Geometry check sheet. Reference: drawing and pictorial views, mm from the part's lowest x, y, z. Give positions to 0.01 mm unless a question says otherwise; leave off trailing zeros. Write each loop counter-clockwise with the first axis right and the second up, starting at its lowest first coordinate (ties: lowest second). Pieces come first, ordered by that corner, then holes. Notation, with made-up numbers: (45, -12) -> (64, -12) arc R21 cw to (64, 25) -> close; hole circle Ø11 at (-12.5, -7.75). An arc over 180 degrees is marked (long way). Write each question's results on one line, items separated by ' | '. Start each with the question number.
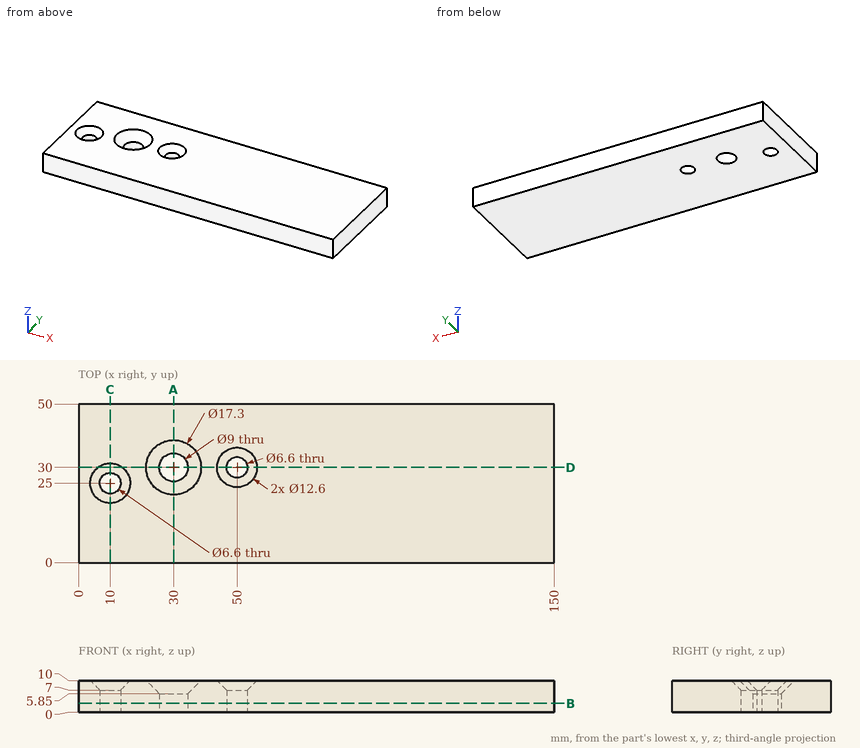
Item 1: Section check B-B on z = 2.75. Record the boundary of the cut face in (x, y).
Item 2: Section check A-A on x = 30. Record the boundary of the cut face in (y, z), then the cut area to 3 significant figures.
Item 3: Section check D-D on y = 30. Count the separate pieces of the cut face and the enclosed holes in it, then the cut area to 3 significant figures.
Item 4: Thickness scan on probe 1 along X at (y, z) = (30, 3.5); probe 2 along Y at (x, z) = (10, 1.5); probe 3 along X at (y, z) = (25, 4.5). Record the ranges inside material, lowest first. Write a range as from..to.
Item 5: Depth check by flat-ended pin: pin 1 Ø5.5 at (x, y) = (30, 30) entering from +Z. Enter the tip coordinate at first touch or a pass-through.
Item 6: Section check C-C on x = 10. Record the boundary of the cut face in (y, z), then the cut area to 3 significant figures.
Check sheet entries:
1) outline: (0, 0) -> (150, 0) -> (150, 50) -> (0, 50) -> close; hole circle Ø6.6 at (10, 25); hole circle Ø9 at (30, 30); hole circle Ø6.6 at (50, 30)
2) outline: (0, 0) -> (25.5, 0) -> (25.5, 5.85) -> (21.35, 10) -> (0, 10) -> close; (34.5, 0) -> (50, 0) -> (50, 10) -> (38.65, 10) -> (34.5, 5.85) -> close | area: 393 mm^2
3) separate pieces: 3 | enclosed holes: 0 | area: 1,310 mm^2
4) probe 1: x = 0..25.5, 34.5..46.7, 53.3..150 | probe 2: y = 0..21.7, 28.3..50 | probe 3: x = 0..6.7, 13.3..150
5) pin 1: passes through
6) outline: (0, 0) -> (21.7, 0) -> (21.7, 7) -> (18.7, 10) -> (0, 10) -> close; (28.3, 0) -> (50, 0) -> (50, 10) -> (31.3, 10) -> (28.3, 7) -> close | area: 425 mm^2
